Here's the drawing with two shaded views (mm, measured from the low corner). I have some questions. A direction names the side the tool comes from. Round coordinates to 2 decimals unless told otherwise and drop trailing zeros. Order: outer loops, then holes, each group sorted by start corner. A loop starts at its lowest first (then second) coordinate and runs counter-clockwise, first axis right, second up. Notation, with made-up numbers: (-26.75, 54.5) -> (16.25, 54.5) arc R21 ccw to (16.25, 61.5) -> close; hole circle Ø11 at (22.25, 50). An arc over 180 degrees is marked (long way). Use a Markdown table: item, result. Add a question column.
Q1. For the marked faces 1 and 2, which set-ups out of +Z, -Z, +X, -X, +Y, -Y let a thin tool reach every point of the face, with its end or its side?
Q2. I need wall thicknesses on line 1 along Z through (x, y) = (1.5, 7); line 2 along X through (y, z) = (13.5, 2.45); line 3 along X through (y, z) = (6.5, 0.6). Which ranges of each line are inside material? Lowest first, please. Write a range as [from, to].
Q3. If we section it at C-C on z = 2.05: List the corners of the cut face in (x, y) for me.
Q4. I'm going to push a flat-ended pin straight in: pin 1 Ø1.5 at (x, z) = (10, 2) entering from -Y. Where does the tip first touch, or does it pass through?
Q5. If we section it at A-A on x = 8: List the corners of the cut face in (y, z) for me.
Q6. If we section it at D-D on z = 3.2: List the corners of the cut face in (x, y) for me.
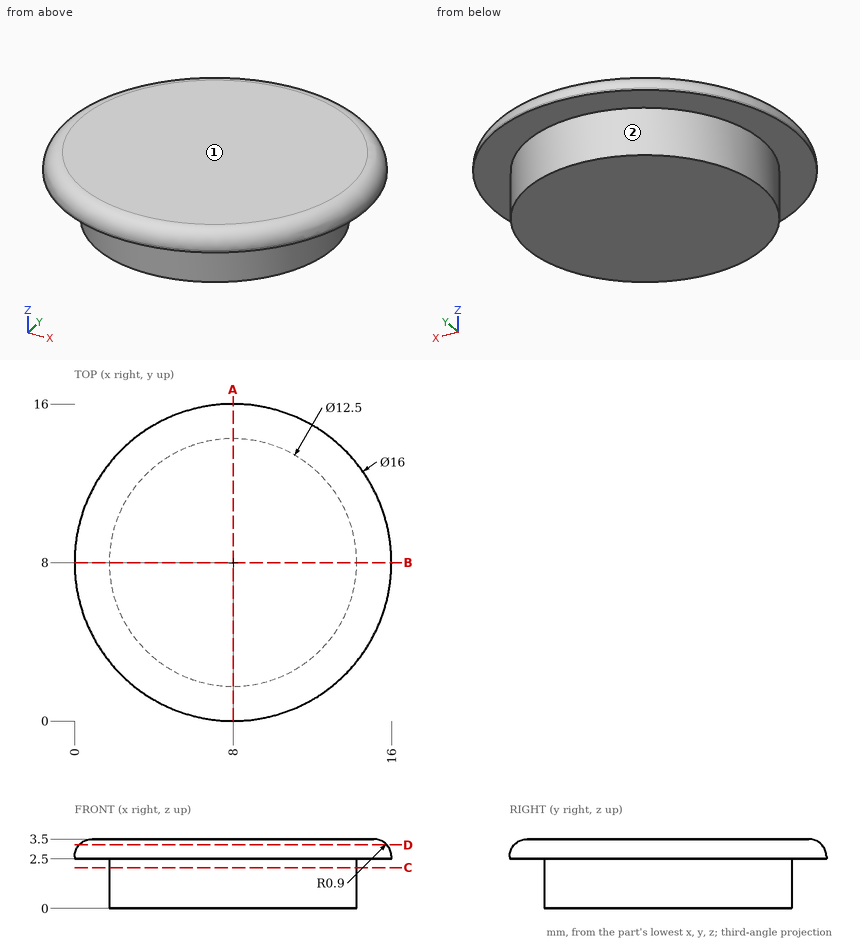
Answer below:
| question | item | result |
|---|---|---|
| 1 | face 1 | +Z, +X, -X, +Y, -Y |
| 1 | face 2 | -Z |
| 2 | line 1 | [2.5, 3.5] |
| 2 | line 2 | [5.03, 10.97] |
| 2 | line 3 | [1.93, 14.07] |
| 3 | outline | circle Ø12.5 at (8, 8) |
| 4 | pin 1 | y = 0.13 |
| 5 | outline | (0, 2.5) -> (1.75, 2.5) -> (1.75, 0) -> (14.25, 0) -> (14.25, 2.5) -> (16, 2.5) -> (16, 2.6) arc R0.9 ccw to (15.1, 3.5) -> (0.9, 3.5) arc R0.9 ccw to (0, 2.6) -> close |
| 6 | outline | circle Ø15.54 at (8, 8) |
